Read the model definition and answer for the solid it produces. Units are mm, in the model's axes. Face numbers are marked on the shaded views. A direction names the side the tool comes from. Round coordinates to 2 decimals unless told otherwise and drop trailing zeros. Order: outer loops, then holes, each group sorted by start corner. A loop starts at its lowest first (then second) coordinate and runs counter-clockwise, first axis right, second up. Notation, with made-up numbers: (13, -19.75) - (67, -19.75) arc R25 ccw to (67, -4.75) - close; hole circle Ø4 at (-28, 87). An arc over 180 degrees is marked (long way). One line per question, with ' | ' between items. Start each with the question number.
1) Straight lines are drawn through the part: line 1 (X direction, y = 2, z = 19.25); line 2 (Y direction, x = 25.5, z = 13.5); line 3 (X direction, y = 9.75, z = 5.25). For each, find the intervals that lie inside material, in ascending order. Write a range as from..to.
2) Flat-ended cylindrical pins translate along their axes: pin 1 (1.5 mm diameter, centred on x = 7, z = 5.5, fed in from +Y); pin 2 (7.5 mm diameter, centred on x = 47.5, z = 13.5, fed in from +Y); pin 3 (0.8 mm diameter, centred on x = 46, z = 7, fed in from +Y); pin 4 (8 mm diameter, centred on y = 12.5, z = 18.5, fed in from -X). Find the tip coordinate at first contact, or state that the pin passes through.
3) The part is cut by section C-C, the plane x = -8. Give the vertices of the cut face in (y, z).
4) The part is cut by section B-B, the plane x = 21. Give the vertices of the cut face in (y, z).
5) The part is cut by section A-A, the plane y = 1.5. Give the vertices of the cut face in (x, z).
6) For the marked faces 1 and 2, determine the directions among +Z, -Z, +X, -X, +Y, -Y from which every point of the face is accessible in a straight line to the end or side of a thin tool.
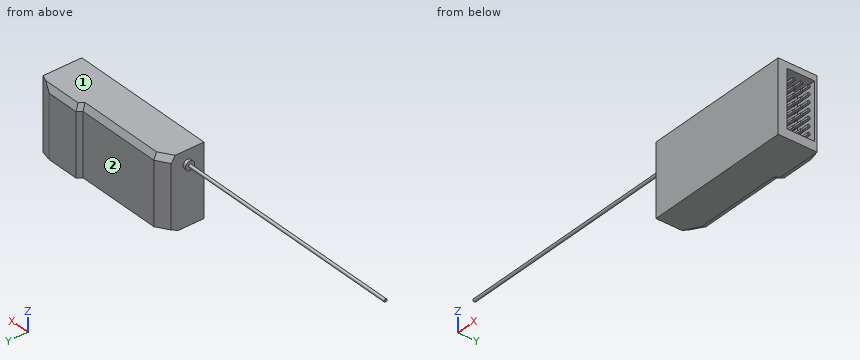
from build123d import *
from OCP.BRepFilletAPI import BRepFilletAPI_MakeChamfer

# Parameters (mm, degrees)
BOSS_EXTRUDE1_DEPTH  = 24
SKETCH2_W            = 19
SKETCH2_H            = 9.2
CUT_EXTRUDE1_DEPTH   = 7
SKETCH3_W            = 0.7
SKETCH3_H            = 0.7
BOSS_EXTRUDE2_DEPTH  = 7
LPATTERN1_COUNT      = 7
LPATTERN1_PITCH      = 2.5
LPATTERN1_COUNT_DIR2 = 3
LPATTERN1_PITCH_DIR2 = 2.5
CHAMFER1_SIZE        = 2
CHAMFER1_SIZE2       = 1.154700538
SKETCH5_R            = 1.5
BOSS_EXTRUDE3_DEPTH  = 1
SKETCH6_R            = 0.5
BOSS_EXTRUDE4_DEPTH  = 80


with BuildPart() as part:
    # Sketch1 → Boss-Extrude1 (new body)
    with BuildSketch(Plane.XY):
        Polygon((0, 0), (0, 11), (4, 13.5), (33, 13.5), (34, 15), (45, 15), (50, 13), (50, 0), align=None)
    extrude(amount=BOSS_EXTRUDE1_DEPTH)

    # Sketch2 → Cut-Extrude1 (cut)
    with BuildSketch(Plane(origin=(50, 0, 0), x_dir=(0, 0, -1), z_dir=(1, 0, 0))):
        with Locations((-12.5, 7.6)):
            Rectangle(SKETCH2_W, SKETCH2_H)
    extrude(amount=-CUT_EXTRUDE1_DEPTH, mode=Mode.SUBTRACT)

    # Sketch3 → Boss-Extrude2 (add)
    with BuildSketch(Plane(origin=(43, 0, 0), x_dir=(0, 0, -1), z_dir=(1, 0, 0))):
        with Locations((-19.65, 5.35)):
            Rectangle(SKETCH3_W, SKETCH3_H)
    boss_extrude2 = extrude(amount=BOSS_EXTRUDE2_DEPTH)

    # LPattern1: Boss-Extrude2 7 × 3
    with Locations(*[(0, j * LPATTERN1_PITCH_DIR2, -i * LPATTERN1_PITCH) for i in range(LPATTERN1_COUNT) for j in range(LPATTERN1_COUNT_DIR2) if (i, j) != (0, 0)]):
        add(boss_extrude2)

    # Chamfer1: one chamfer whose edges measure the first distance from different faces: ONE call of the kernel's chamfer builder (chamfer() names one face for all edges)
    chamfer1_edges_1 = [part.edges().sort_by_distance(p)[0] for p in [
        (39.5, 15, 0),
        (33.5, 14.25, 0),
        (18.5, 13.5, 0),
        (2, 12.25, 0),
    ]]
    chamfer1_side_1 = [part.faces().sort_by_distance(p)[0] for p in [
        (25.603358705, 6.920985864, 0),
    ]]
    chamfer1_edges_2 = [part.edges().sort_by_distance(p)[0] for p in [
        (39.5, 15, 24),
    ]]
    chamfer1_side_2 = [part.faces().sort_by_distance(p)[0] for p in [
        (39.5, 15, 12),
    ]]
    chamfer1_edges_3 = [part.edges().sort_by_distance(p)[0] for p in [
        (33.5, 14.25, 24),
    ]]
    chamfer1_side_3 = [part.faces().sort_by_distance(p)[0] for p in [
        (33.5, 14.25, 12),
    ]]
    chamfer1_edges_4 = [part.edges().sort_by_distance(p)[0] for p in [
        (2, 12.25, 24),
    ]]
    chamfer1_side_4 = [part.faces().sort_by_distance(p)[0] for p in [
        (2, 12.25, 12),
    ]]
    chamfer1_edges_5 = [part.edges().sort_by_distance(p)[0] for p in [
        (18.5, 13.5, 24),
    ]]
    chamfer1_side_5 = [part.faces().sort_by_distance(p)[0] for p in [
        (18.5, 13.5, 12),
    ]]
    chamfer1 = BRepFilletAPI_MakeChamfer(part.part.solid().wrapped)
    for e in chamfer1_edges_1:
        chamfer1.Add(CHAMFER1_SIZE, CHAMFER1_SIZE2, e.wrapped, chamfer1_side_1[0].wrapped)  # the first distance lies on this face
    for e in chamfer1_edges_2:
        chamfer1.Add(CHAMFER1_SIZE, CHAMFER1_SIZE2, e.wrapped, chamfer1_side_2[0].wrapped)  # the first distance lies on this face
    for e in chamfer1_edges_3:
        chamfer1.Add(CHAMFER1_SIZE, CHAMFER1_SIZE2, e.wrapped, chamfer1_side_3[0].wrapped)  # the first distance lies on this face
    for e in chamfer1_edges_4:
        chamfer1.Add(CHAMFER1_SIZE, CHAMFER1_SIZE2, e.wrapped, chamfer1_side_4[0].wrapped)  # the first distance lies on this face
    for e in chamfer1_edges_5:
        chamfer1.Add(CHAMFER1_SIZE, CHAMFER1_SIZE2, e.wrapped, chamfer1_side_5[0].wrapped)  # the first distance lies on this face
    add(Compound.cast(chamfer1.Shape()), mode=Mode.REPLACE)

    # Sketch5 → Boss-Extrude3 (add)
    with BuildSketch(Plane.ZY):
        with Locations(Location((19.5, 5.5, 0), (0, 0, 180))):
            Circle(SKETCH5_R)
    extrude(amount=BOSS_EXTRUDE3_DEPTH)

    # Sketch6 → Boss-Extrude4 (add)
    with BuildSketch(Plane.ZY.offset(1)):
        with Locations((19.5, 5.5)):
            Circle(SKETCH6_R)
    extrude(amount=BOSS_EXTRUDE4_DEPTH)


solid = part.part
Values:
1) line 1: x = 0..50 | line 2: y = 0..13.5 | line 3: x = 0..43
2) pin 1: stops at y = 13.5 | pin 2: stops at y = 15 | pin 3: stops at y = 14.76 | pin 4: stops at x = 0
3) outline: circle Ø1 at (5.5, 19.5)
4) outline: (0, 0) - (11.5, 0) - (13.5, 1.15) - (13.5, 22) - (12.35, 24) - (0, 24) - close
5) outline: (0, 0) - (50, 0) - (50, 24) - (0, 24) - close
6) face 1: +Z, +X, -X, +Y, -Y | face 2: +Z, -Z, -X, +Y
